Here's the drawing with two shaded views (mm, measured from the low corner). I have some questions. A direction names the side the tool comes from. Round coordinates to 2 decimals unless told otherwise and drop trailing zeros. Order: outer loops, then holes, each group sorted by start corner. A loop starts at its lowest first (then second) coordinate and runs counter-clockwise, first axis right, second up. Notation, with made-up numbers: (-21, 65.5) -> (35, 65.5) arc R21 cw to (35, 79.5) -> close; hole circle Ø3 at (32, 2.25). An arc over 180 degrees is marked (long way). Answer in a Markdown table with one row per item.
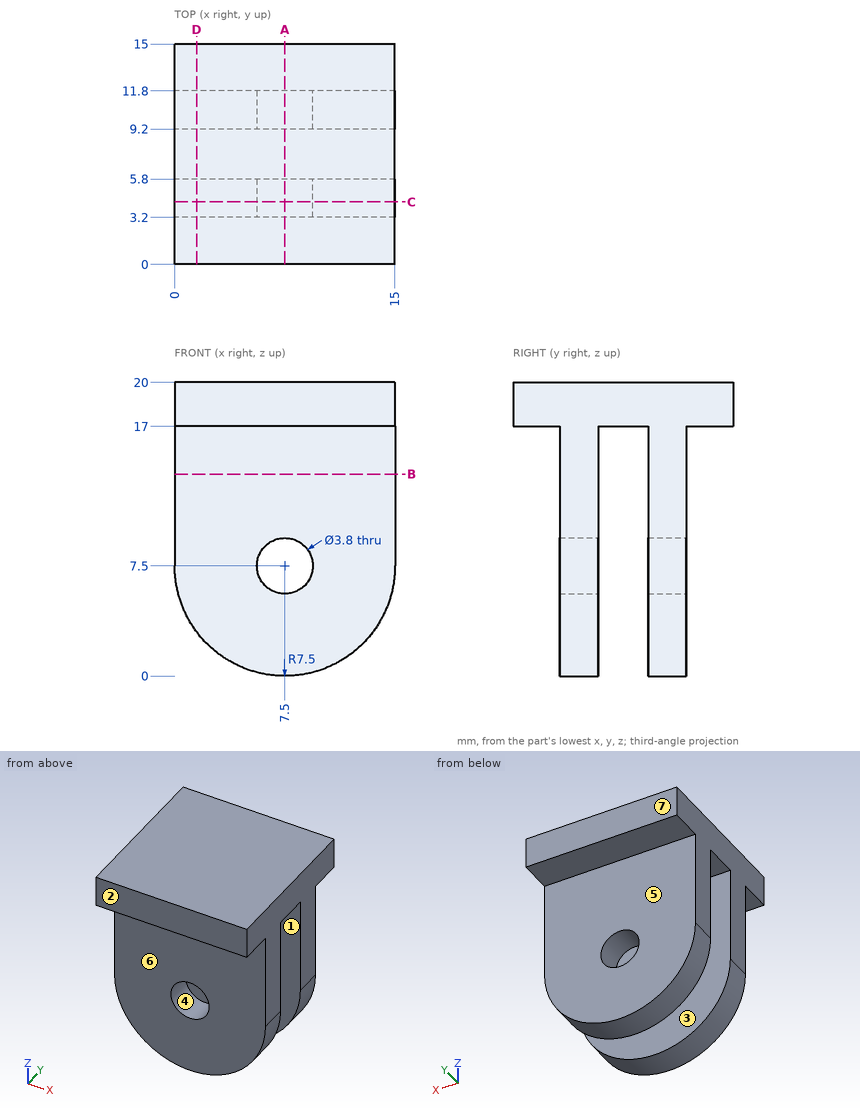
1. For the marked faces 5, 6 and 7, which set-ups out of +Z, -Z, +X, -X, +Y, -Y let a thin tool reach every point of the face, with its end or its side?
Numbers:
| item | result |
|---|---|
| face 5 | -Z, +X, -X, +Y |
| face 6 | -Z, +X, -X, -Y |
| face 7 | +Z, -Z, +X, -X, +Y |
2. Suppose I cut it at B-B on z = 13.75. Write out the boundary of the cut face in (x, y), then the cut area to 3 significant figures.
Numbers:
| item | result |
|---|---|
| outline | (0, 3.2) -> (15, 3.2) -> (15, 5.8) -> (0, 5.8) -> close; (0, 9.2) -> (15, 9.2) -> (15, 11.8) -> (0, 11.8) -> close |
| area | 78.0 mm2 |
3. Suppose I cut it at C-C on y = 4.25. Write out the boundary of the cut face in (x, z), then the cut area to 3 significant figures.
Numbers:
| item | result |
|---|---|
| outline | (0, 7.5) arc R7.5 ccw to (15, 7.5) -> (15, 20) -> (0, 20) -> close; hole circle Ø3.8 at (7.5, 7.5) |
| area | 265 mm2 |
4. Please list where these lines run through material, in increasing order: line 1 along Z through (x, y) = (7.5, 10.1); line 2 along Y through (x, z) = (2, 7); line 3 along Z through (x, y) = (13.75, 6.5).
Numbers:
| item | result |
|---|---|
| line 1 | z = 0 to 5.6, 9.4 to 20 |
| line 2 | y = 3.2 to 5.8, 9.2 to 11.8 |
| line 3 | z = 17 to 20 |
5. We'd pull the mould along Y, two halves only. Please class the marked faces 1, 2, 3 and 4: released by +Y, released by -Y, zero draft, split by the parting line, or undercut.
Numbers:
| item | result |
|---|---|
| face 1 | undercut |
| face 2 | released by -Y |
| face 3 | undercut |
| face 4 | zero draft |
6. Suppose I cut it at A-A on x = 7.5. Write out the boundary of the cut face in (y, z), then the cut area to 3 significant figures.
Numbers:
| item | result |
|---|---|
| outline | (0, 17) -> (3.2, 17) -> (3.2, 9.4) -> (5.8, 9.4) -> (5.8, 17) -> (9.2, 17) -> (9.2, 9.4) -> (11.8, 9.4) -> (11.8, 17) -> (15, 17) -> (15, 20) -> (0, 20) -> close; (3.2, 0) -> (5.8, 0) -> (5.8, 5.6) -> (3.2, 5.6) -> close; (9.2, 0) -> (11.8, 0) -> (11.8, 5.6) -> (9.2, 5.6) -> close |
| area | 114 mm2 |
7. For pin 1 Ø3.5 at (x, y) = (9.5, 2) entering from -Z; pin 2 Ø3 at (x, z) = (6, 2.5) entering from -Y; pin 3 Ø4.5 at (x, z) = (5.5, 12) entering from +Y, each with a flat end and sliding along its axis, tell me the tip position at first contact or that it passes through.
Numbers:
| item | result |
|---|---|
| pin 1 | stops at z = 0.04 |
| pin 2 | stops at y = 3.2 |
| pin 3 | stops at y = 11.8 |
8. Suppose I cut it at D-D on x = 1.5. Write out the boundary of the cut face in (y, z).
Numbers:
| item | result |
|---|---|
| outline | (0, 17) -> (3.2, 17) -> (3.2, 3) -> (5.8, 3) -> (5.8, 17) -> (9.2, 17) -> (9.2, 3) -> (11.8, 3) -> (11.8, 17) -> (15, 17) -> (15, 20) -> (0, 20) -> close |
